Can you work these out from the model? Positions are in its coordinate system, mm. Face numbers are marked on the shaded views. A direction names the side the tool comes from. Coordinates: 2 decimals unless noted, no trailing zeros. Write each loop counter-clockwise with the first axis right and the second up, starting at its lowest first coordinate (ties: lowest second). Pieces come first, ordered by that corner, then holes. Notation, with made-up numbers: M 88,55.5 L 92,55.5 A11 ccw 92,60.5 Z; hole C 34,50 d3. An arc over 180 degrees is marked long. Answer as a JSON object with one key per item and string values. Group by question number.
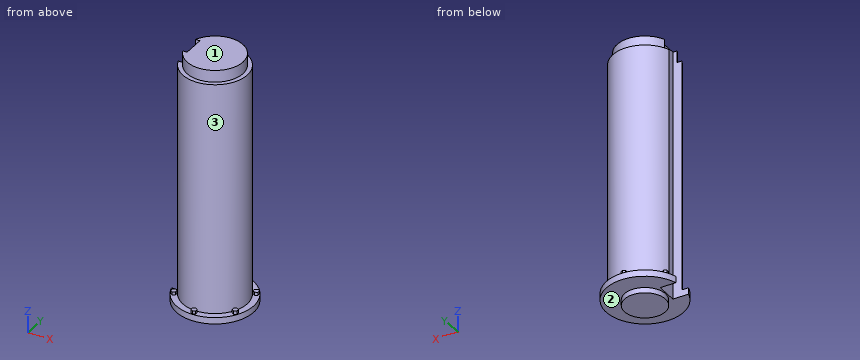
from build123d import *

# Parameters (mm, degrees)
SKETCH_R           = 18
PAD_DEPTH          = 3
SKETCH001_R        = 15
PAD001_DEPTH       = 108
SKETCH002_R        = 9.5
PAD002_DEPTH       = 2.5
SKETCH003_R        = 13
PAD003_DEPTH       = 5.5
PAD004_DEPTH       = 1.5
POLARPATTERN_COUNT = 6
SKETCH009_W        = 8
SKETCH009_H        = 10
POCKET_DEPTH       = 118


with BuildPart() as part:
    # Sketch → Pad (new body)
    with BuildSketch(Plane.XY):
        Circle(SKETCH_R)
    extrude(amount=PAD_DEPTH)

    # Sketch001 (on Face3 of Pad) → Pad001 (join)
    with BuildSketch(Plane.XY.offset(3)):
        Circle(SKETCH001_R)
    extrude(amount=PAD001_DEPTH)

    # Sketch002 (on Face2 of Pad001) → Pad002 (join)
    with BuildSketch(Plane(origin=(0, 0, 0), x_dir=(1, 0, 0), z_dir=(0, 0, -1))):
        Circle(SKETCH002_R)
    extrude(amount=PAD002_DEPTH)

    # Sketch003 (on Face7 of Pad002) → Pad003 (join)
    with BuildSketch(Plane.XY.offset(111)):
        Circle(SKETCH003_R)
    extrude(amount=PAD003_DEPTH)

    # Sketch008 (on Face3 of Pad003) → Pad004 (join)
    with BuildSketch(Plane.XY.offset(3)):
        Polygon((-1.11579, 17.121659), (-0.012041, 17.758909), (1.091708, 17.121659), (1.091708, 15.84716), (-0.012041, 15.209911), (-1.11579, 15.84716), align=None)
    pad004 = extrude(amount=PAD004_DEPTH)

    # PolarPattern: Pad004 ×6 about axis
    polarpattern_axis = Axis((0, 0, 3), (0, 0, 1))
    for i in range(1, POLARPATTERN_COUNT):
        add(pad004.rotate(polarpattern_axis, i * 360 / POLARPATTERN_COUNT))

    # Sketch009 (on Face2 of PolarPattern) → Pocket (cut)
    with BuildSketch(Plane(origin=(0, 0, 0), x_dir=(1, 0, 0), z_dir=(0, 0, -1))):
        with Locations((-14, 0)):
            Rectangle(SKETCH009_W, SKETCH009_H)
    extrude(amount=-POCKET_DEPTH, mode=Mode.SUBTRACT)


solid = part.part
Q1. On a 3-axis mill with a long thin cutter (end or side, diameter ignored), from which of +Z, -Z, +X, -X, +Y, -Y can I reach the whole of each face in a straight line? I mean the marked faces 1, 2 and 3. Say none if no direction works.
Q2. If we section it at D-D on x = 6.5: List the corners of the cut face in (y, z) for me.
Q3. If we section it at B-B on x = -5.5: List the corners of the cut face in (y, z) for me.
Q4. If we section it at C-C on z = 44: List the corners of the cut face in (x, y) for me, and give its area (3 significant figures).
Q5. Please list where these lines run through material, in increasing order: L1, parallel to Z at x = 12, y = -8.5; L2, parallel to Z at x = 16, y = 2; L3, parallel to Y at x = 4.5, z = 51.5.
Q6. If we section it at A-A on y = 0: List the corners of the cut face in (x, z) for me, and give its area (3 significant figures).
Q7. Will these pins go through, and if not, where does the flat tip stop? pin 1 (12 mm diameter, centred on x = -12.5, y = 6, fed in from -Z); pin 2 (2 mm diameter, centred on x = -1.5, z = 54.5, fed in from -Y); pin 3 (2.5 mm diameter, centred on x = -13.5, y = 7.5, fed in from +Z); pin 4 (6 mm diameter, centred on x = 2.5, z = 11, fed in from +Y).
Reply:
{
 "1": {"face 1": "+Z, +X, -X, +Y, -Y", "face 2": "-Z", "face 3": "+Z"},
 "2": {"outline": "M -16.79,0 L -6.93,0 L -6.93,-2.5 L 6.93,-2.5 L 6.93,0 L 16.79,0 L 16.79,3 L 13.52,3 L 13.52,111 L 11.26,111 L 11.26,116.5 L -11.26,116.5 L -11.26,111 L -13.52,111 L -13.52,3 L -16.79,3 Z"},
 "3": {"outline": "M -17.14,0 L -7.75,0 L -7.75,-2.5 L 7.75,-2.5 L 7.75,0 L 17.14,0 L 17.14,3 L 13.96,3 L 13.96,111 L 11.78,111 L 11.78,116.5 L -11.78,116.5 L -11.78,111 L -13.96,111 L -13.96,3 L -17.14,3 Z"},
 "4": {"outline": "M -14.14,-5 A15 ccw long -14.14,5 L -10,5 L -10,-5 Z", "area": "660 mm^2"},
 "5": {"L1": "0 to 111", "L2": "0 to 3", "L3": "-14.31 to 14.31"},
 "6": {"outline": "M -10,0 L -9.5,0 L -9.5,-2.5 L 9.5,-2.5 L 9.5,0 L 18,0 L 18,3 L 15,3 L 15,111 L 13,111 L 13,116.5 L -10,116.5 Z", "area": "2,960 mm^2"},
 "7": {"pin 1": "z = -2.5", "pin 2": "y = -14.99", "pin 3": "z = 111", "pin 4": "y = 15"}
}
